Autodesk Inventor part; units mm, degrees
ref_plane "YZ Plane" through (0, 0, 0) normal (1, 0, 0) x (0, 1, 0)
ref_plane "XZ Plane" through (0, 0, 0) normal (0, 1, 0) x (-1, 0, 0)
ref_plane "XY Plane" through (0, 0, 0) normal (0, 0, 1) x (1, 0, 0)
sketch "Sketch1" plane through (0, 0, 0) normal (0, 1, 0) x (-1, 0, 0)
  line L0 (0, 0) -> (596.9, 0)
  line L1 (596.9, 0) -> (596.9, -571.5)
  line L2 (596.9, -571.5) -> (0, -571.5)
  line L3 (0, -571.5) -> (0, 0)
  line L4 (596.9, 0) -> (0, 0)
  line L5 (0, 0) -> (0, -38.1)
  line L6 (0, -38.1) -> (596.9, -38.1)
  line L7 (596.9, -38.1) -> (596.9, 0)
  line L8 (25.4, -38.1) -> (571.5, -38.1)
  line L9 (571.5, -38.1) -> (571.5, -88.9)
  line L10 (571.5, -88.9) -> (25.4, -88.9)
  line L11 (25.4, -88.9) -> (25.4, -38.1)
  line L12 (400.05, -88.9) -> (222.25, -88.9)
  line L13 (222.25, -88.9) -> (222.25, -266.7)
  line L14 (222.25, -266.7) -> (400.05, -266.7)
  line L15 (400.05, -266.7) -> (400.05, -88.9)
  line L16 (596.9, -266.7) -> (0, -266.7)
  line L17 (0, -266.7) -> (0, -342.9)
  line L18 (0, -342.9) -> (596.9, -342.9)
  line L19 (596.9, -342.9) -> (596.9, -266.7)
  line L20 (568.9457, -342.9) -> (52.0133, -342.9)
  line L21 (52.0133, -419.1) -> (568.9457, -419.1)
  line L22 (596.9, -419.1) -> (0, -419.1)
  line L23 (0, -419.1) -> (0, -571.5)
  line L24 (0, -571.5) -> (596.9, -571.5)
  line L25 (596.9, -571.5) -> (596.9, -419.1)
  line L26 (571.5, -266.7) -> (25.4, -266.7)
  line L27 (25.4, -266.7) -> (25.4, -342.9)
  line L28 (25.4, -342.9) -> (571.5, -342.9)
  line L29 (571.5, -342.9) -> (571.5, -266.7)
  line L30 (552.45, -419.1) -> (44.45, -419.1)
  line L31 (44.45, -419.1) -> (44.45, -508)
  line L32 (44.45, -508) -> (552.45, -508)
  line L33 (552.45, -508) -> (552.45, -419.1)
  line L34 (596.9, -571.5) -> (0, -571.5)
  line L35 (0, -571.5) -> (0, -482.6)
  line L36 (0, -482.6) -> (596.9, -482.6)
  line L37 (596.9, -482.6) -> (596.9, -571.5)
  dimension "d0" = 596.9
  dimension "d1" = 571.5
  dimension "d2" = 38.1
  dimension "d3" = 50.8
  dimension "d4" = 177.8
  dimension "d6" = 76.2
  dimension "d7" = 76.2
  dimension "d8" = 88.9
  dimension "d9" = 88.9
  dimension "d10" = 44.45
  dimension "d11" = 44.45
  dimension "d12" = 25.4
  dimension "d13" = 25.4
  dimension "d14" = 177.8
  dimension "d15" = 196.85
  dimension "d16" = 25.4
  dimension "d17" = 25.4
extrude "Extrusion1" add sketch "Sketch1" along normal blind 6.35 contours L0 L1 L6 L3 | L6 L9 L10 L11 | L1 L18 L29 L16 | L18 L1 L22 L21 L3 | L16 L14 L29 L18 L27 | L13 L10 L15 L14 | L36 L31 L32 L33 L1 L2 L3 | L22 L21 L33 L36 L31 | L36 L33 L32 L31
properties part number "ElectricalBoard.ver2-1111-2020"
The listing builds one solid part. Answer for the finished solid, in the listing's coordinates (mm). Give positions to 0.01 mm unless a question says otherwise; leave off trailing zeros. Write each loop counter-clockwise with the first axis right and the second up, starting at its lowest first coordinate (ties: lowest second). Pieces come first, ordered by that corner, then holes.
Item 1: Flat-ended cylindrical pins translate along their axes: P1, Ø1.9, axis at x = -507.5, y = 2.5, coming from the +Z side; P2, Ø3, axis at y = 3.5, z = -61, coming from the +X side; P3, Ø3, axis at y = 3.5, z = -71.5, coming from the -X side; P4, Ø3, axis at y = 3, z = -176, coming from the -X side. Find the tip coordinate at first contact, or state that the pin passes through.
Item 2: Section A-A, the plane x = -529 is taken. Write down the section's boundary in (y, z), plus the area to 3 significant figures.
Item 3: Section C-C, the plane z = -58 is taken. Write down the section's boundary in (x, y), plus the area to 3 significant figures.
Item 4: Section D-D, the plane z = -473.5 is taken. Write down the section's boundary in (x, y), plus the area to 3 significant figures.
Item 5: Section B-B, the plane y = 2.25 is taken. Write down the section's boundary in (x, z), plus the area to 3 significant figures.
Item 6: Find the intervals of material crossed by line 1 along Z through (x, y) = (-27, 2.25); line 2 along Z through (x, y) = (-130, 6.25); line 3 along X through (y, z) = (4, -329.5), in increasing order.
Completed:
1. P1: stops at z = 0
1. P2: stops at x = -25.4
1. P3: stops at x = -571.5
1. P4: stops at x = -400.05
2. outline: (0, -571.5) - (6.35, -571.5) - (6.35, -266.7) - (0, -266.7) - close; (0, -88.9) - (6.35, -88.9) - (6.35, 0) - (0, 0) - close
2. area: 2,500 mm2
3. outline: (-571.5, 0) - (-25.4, 0) - (-25.4, 6.35) - (-571.5, 6.35) - close
3. area: 3,470 mm2
4. outline: (-552.45, 0) - (-44.45, 0) - (-44.45, 6.35) - (-552.45, 6.35) - close
4. area: 3,230 mm2
5. outline: (-596.9, -571.5) - (0, -571.5) - (0, -482.6) - (-44.45, -482.6) - (-44.45, -419.1) - (0, -419.1) - (0, -342.9) - (-25.4, -342.9) - (-25.4, -266.7) - (-222.25, -266.7) - (-222.25, -88.9) - (-25.4, -88.9) - (-25.4, -38.1) - (0, -38.1) - (0, 0) - (-596.9, 0) - (-596.9, -38.1) - (-571.5, -38.1) - (-571.5, -88.9) - (-400.05, -88.9) - (-400.05, -266.7) - (-596.9, -266.7) - (-596.9, -419.1) - (-552.45, -419.1) - (-552.45, -482.6) - (-596.9, -482.6) - close
5. area: 256,000 mm2
6. line 1: z = -571.5 to -482.6, -419.1 to -266.7, -88.9 to 0
6. line 2: z = -571.5 to -266.7, -88.9 to 0
6. line 3: x = -596.9 to -25.4
